from build123d import *

# Parameters (mm, degrees)
SKETCH1_R             = 3.9
SKETCH1_R_2           = 1.5
BOSS_EXTRUDE1_DEPTH   = 13.361552014
BOSS_EXTRUDE1_2_DEPTH = 13.361552014
BOSS_EXTRUDE1_3_DEPTH = 13.361552014
BOSS_EXTRUDE1_4_DEPTH = 13.361552014
BOSS_EXTRUDE2_START   = 5.161552
SKETCH2_R             = 3.9
SKETCH2_R_2           = 9.3
BOSS_EXTRUDE2_DEPTH   = 10
CUT_EXTRUDE1_DEPTH    = 25
CUT_EXTRUDE2_DEPTH    = 72.711443105
SKETCH5_W             = 10
SKETCH5_H             = 10
SKETCH5_R             = 2
BOSS_EXTRUDE3_DEPTH   = 10


with BuildPart() as part:
    # Sketch1 → Boss-Extrude1 (new body)
    with BuildSketch(Plane.XY):
        with Locations(Location((-49, 7.83595021, 0), (0, 0, 90))):
            Circle(SKETCH1_R)
        with Locations(Location((-49, 7.83595021, 0), (0, 0, 90))):
            Circle(SKETCH1_R_2, mode=Mode.SUBTRACT)
    extrude(amount=BOSS_EXTRUDE1_DEPTH)



with BuildPart() as body_2:
    # Sketch1 → Boss-Extrude1 2 (new body)
    with BuildSketch(Plane.XY):
        with Locations(Location((-49, 35.83595021, 0), (0, 0, 90))):
            Circle(SKETCH1_R)
        with Locations(Location((-49, 35.83595021, 0), (0, 0, 90))):
            Circle(SKETCH1_R_2, mode=Mode.SUBTRACT)
    extrude(amount=BOSS_EXTRUDE1_2_DEPTH)


with BuildPart() as body_3:
    # Sketch1 → Boss-Extrude1 3 (new body)
    with BuildSketch(Plane.XY):
        with Locations(Location((-9, 35.83595021, 0), (0, 0, 90))):
            Circle(SKETCH1_R)
        with Locations(Location((-9, 35.83595021, 0), (0, 0, 90))):
            Circle(SKETCH1_R_2, mode=Mode.SUBTRACT)
    extrude(amount=BOSS_EXTRUDE1_3_DEPTH)


with BuildPart() as body_4:
    # Sketch1 → Boss-Extrude1 4 (new body)
    with BuildSketch(Plane.XY):
        with Locations(Location((-9, 7.83595021, 0), (0, 0, 90))):
            Circle(SKETCH1_R)
        with Locations(Location((-9, 7.83595021, 0), (0, 0, 90))):
            Circle(SKETCH1_R_2, mode=Mode.SUBTRACT)
    extrude(amount=BOSS_EXTRUDE1_4_DEPTH)


with BuildPart() as part_1:
    add(part.part)

    add(body_2.part)  # Boss-Extrude2 merges body 2

    add(body_3.part)  # Boss-Extrude2 merges body 3

    add(body_4.part)  # Boss-Extrude2 merges body 4
    # Sketch2 → Boss-Extrude2 (add)
    with BuildSketch(Plane.XY.offset(-1.8).offset(BOSS_EXTRUDE2_START)):
        Polygon((-58, 1.83595021), (0, 1.83595021), (0, 5.290014366), (0, 38.441339865), (0, 41.83595021), (-58, 41.83595021), align=None)
        with Locations(Location((-9, 35.83595021, 0), (0, 0, 90))):
            Circle(SKETCH2_R, mode=Mode.SUBTRACT)
        with Locations(Location((-49, 7.83595021, 0), (0, 0, 270))):
            Circle(SKETCH2_R, mode=Mode.SUBTRACT)
        with Locations(Location((-38.5, 21.83595021, 0), (0, 0, 90))):
            Circle(SKETCH2_R_2, mode=Mode.SUBTRACT)
        with Locations(Location((-49, 35.83595021, 0), (0, 0, 90))):
            Circle(SKETCH2_R, mode=Mode.SUBTRACT)
        with Locations(Location((-9, 7.83595021, 0), (0, 0, 90))):
            Circle(SKETCH2_R, mode=Mode.SUBTRACT)
    extrude(amount=BOSS_EXTRUDE2_DEPTH)

    # Sketch4 → Cut-Extrude1 (cut)
    with BuildSketch(Plane(origin=(0, 41.83595021, 0), x_dir=(1, 0, 0), z_dir=(0, 1, 0))):
        with BuildLine():
            ThreePointArc((-23, -8.361552014), (-20, -11.361552014), (-17, -8.361552014))
            Line((-17, -8.361552014), (-18, -8.361552014))
            ThreePointArc((-18, -8.361552014), (-20, -10.361552014), (-22, -8.361552014))
            Line((-22, -8.361552014), (-23, -8.361552014))
        make_face()
        with BuildLine():
            Line((-18, -8.361552014), (-17, -8.361552014))
            ThreePointArc((-17, -8.361552014), (-20, -5.361552014), (-23, -8.361552014))
            Line((-23, -8.361552014), (-22, -8.361552014))
            ThreePointArc((-22, -8.361552014), (-20, -6.361552014), (-18, -8.361552014))
        make_face()
        with BuildLine():
            ThreePointArc((-22, -8.361552014), (-20, -10.361552014), (-18, -8.361552014))
            Line((-18, -8.361552014), (-22, -8.361552014))
        make_face()
        with BuildLine():
            Line((-22, -8.361552014), (-18, -8.361552014))
            ThreePointArc((-18, -8.361552014), (-20, -6.361552014), (-22, -8.361552014))
        make_face()
    extrude(amount=-CUT_EXTRUDE1_DEPTH, mode=Mode.SUBTRACT)

    # Sketch4<3> → Cut-Extrude2 (cut, through all)
    with BuildSketch(Plane(origin=(0, 41.83595021, 0), x_dir=(1, 0, 0), z_dir=(0, 1, 0))):
        with BuildLine():
            ThreePointArc((-22, -8.361552014), (-20, -10.361552014), (-18, -8.361552014))
            Line((-18, -8.361552014), (-22, -8.361552014))
        make_face()
        with BuildLine():
            Line((-22, -8.361552014), (-18, -8.361552014))
            ThreePointArc((-18, -8.361552014), (-20, -6.361552014), (-22, -8.361552014))
        make_face()
    extrude(amount=-CUT_EXTRUDE2_DEPTH, mode=Mode.SUBTRACT)

    # Sketch5 → Boss-Extrude3 (add)
    with BuildSketch(Plane(origin=(0, 1.83595021, 0), x_dir=(1, 0, 0), z_dir=(0, 1, 0))):
        with Locations((-63, -8.361552014)):
            Rectangle(SKETCH5_W, SKETCH5_H)
        with Locations(Location((-63, -8.361552014, 0), (0, 0, 180))):
            Circle(SKETCH5_R, mode=Mode.SUBTRACT)
    extrude(amount=BOSS_EXTRUDE3_DEPTH)


solid = part_1.part
Could you check a few things on this model? Use its own coordinates, in mm. A direction names the side the tool comes from. Give positions to 0.01 mm unless a question says otherwise; leave off trailing zeros. Write each loop counter-clockwise with the first axis right and the second up, starting at its lowest first coordinate (ties: lowest second). Pieces come first, ordered by that corner, then holes. Notation, with made-up numbers: (6.25, 44) -> (46.25, 44) arc R32 ccw to (46.25, 80) -> close; hole circle Ø2 at (-33.5, 21.25). An arc over 180 degrees is marked (long way). Answer as a JSON object with one key per item and string values.
Q1. Will these pins go through, and if not, where does the flat tip stop? pin 1 Ø20 at (x, y) = (-33.5, 17) entering from -Z; pin 2 Ø5 at (x, z) = (-63, 8.36) entering from +Y; pin 3 Ø1 at (y, z) = (29.5, 9.5) entering from -X.
Taken from the geometry:
{"pin 1": "stops at z = 3.36", "pin 2": "stops at y = 11.84", "pin 3": "stops at x = -58"}
Q2. Suppose I cut it at B-B on x = -38.5. Write out the boundary of the cut face in (y, z).
Taken from the geometry:
{"outline": "(1.84, 3.36) -> (12.54, 3.36) -> (12.54, 13.36) -> (1.84, 13.36) -> close; (31.14, 3.36) -> (41.84, 3.36) -> (41.84, 13.36) -> (31.14, 13.36) -> close"}
Q3. Suppose I cut it at C-C on z = 4.5. Write out the boundary of the cut face in (x, y), then the cut area to 3 significant figures.
Taken from the geometry:
{"outline": "(-68, 1.84) -> (0, 1.84) -> (0, 41.84) -> (-58, 41.84) -> (-58, 11.84) -> (-68, 11.84) -> close; hole circle Ø3 at (-49, 7.84); hole circle Ø3 at (-49, 35.84); hole circle Ø18.6 at (-38.5, 21.84); hole circle Ø3 at (-9, 7.84); hole circle Ø3 at (-9, 35.84)", "area": "2,120 mm²"}
Q4. Which directions (+Z, -Z, +X, -X, +Y, -Y) give clear straight access to the entire face, cutting with the end or side of a thin tool? Please do faces 1 (the cylindrical face through (-8.087, 6.646, 6.587)), 2 (the flat face through (-58, 27, 8)), 3 (the cylindrical face through (-50.171, 39.556, 1.657)).
Taken from the geometry:
{"face 1": "+Z, -Z", "face 2": "+Z, -Z, -X, +Y", "face 3": "-Z"}
Q5. Suppose I cut it at A-A on z = 1. Write out the boundary of the cut face in (x, y).
Taken from the geometry:
{"outline": "circle Ø7.8 at (-49, 7.84); circle Ø7.8 at (-49, 35.84); circle Ø7.8 at (-9, 7.84); circle Ø7.8 at (-9, 35.84); hole circle Ø3 at (-49, 7.84); hole circle Ø3 at (-49, 35.84); hole circle Ø3 at (-9, 7.84); hole circle Ø3 at (-9, 35.84)"}
Q6. We'd pull the mould along Y, two halves only. Please class faces 4 (the flat face through (-20, 16.836, 6)), 5 (the flat face through (0, 22, 8)), 6 (the cylindrical face through (-52.867, 7.328, 1.657)): released by +Y, released by -Y, zero draft, split by the parting line, or undercut.
Taken from the geometry:
{"face 4": "released by +Y", "face 5": "zero draft", "face 6": "undercut"}
Q7. Please list where these lines run through material, in increasing order: L1, parallel to X at y = 14, z = 9.5; L2, parallel to X at y = 9, z = 4.75; L3, parallel to Z at x = -63, y = 8.
Taken from the geometry:
{"L1": "x = -58 to -43.51, -33.49 to -21.64, -18.36 to 0", "L2": "x = -68 to -49.95, -48.05 to -9.95, -8.05 to 0", "L3": "z = 3.36 to 6.36, 10.36 to 13.36"}
Q8. Suppose I cut it at D-D on x = -49. Write out the boundary of the cut face in (y, z), then the cut area to 3 significant figures.
Taken from the geometry:
{"outline": "(1.84, 3.36) -> (3.94, 3.36) -> (3.94, 0) -> (6.34, 0) -> (6.34, 13.36) -> (1.84, 13.36) -> close; (9.34, 0) -> (11.74, 0) -> (11.74, 3.36) -> (31.94, 3.36) -> (31.94, 0) -> (34.34, 0) -> (34.34, 13.36) -> (9.34, 13.36) -> close; (37.34, 0) -> (39.74, 0) -> (39.74, 3.36) -> (41.84, 3.36) -> (41.84, 13.36) -> (37.34, 13.36) -> close", "area": "372 mm²"}
